Input: part model. Units: mm. Frame: model coordinates. Face numbers are marked on the shaded views. A direction names the side the tool comes from. Coordinates: 2 decimals unless noted, no trailing zeros. Loops run counter-clockwise (first coordinate to the right, second up) from the corner with the lowest first, then second, coordinate; pieces in that order, holes last. Notation, with made-up numbers: (29, 13.25) - (62, 13.25) arc R22 ccw to (62, 35.25) - close; hole circle Ø11 at (0.5, 8). An arc over 180 degrees is marked (long way). Use one line per item in the form item = value.
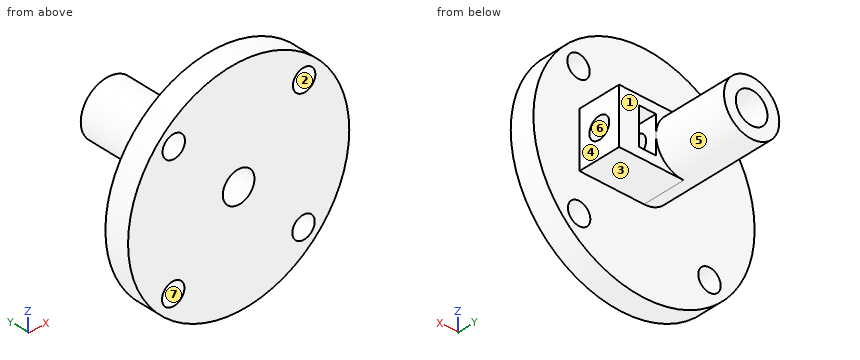
from build123d import *

# Parameters (mm, degrees)
SKETCH1_R           = 18
BOSS_EXTRUDE1_DEPTH = 4
SKETCH2_R           = 1.825
SKETCH2_R_2         = 2.575
CUT_EXTRUDE1_DEPTH  = 26.768197453
BOSS_EXTRUDE2_START = 19
SKETCH3_R           = 4.5
SKETCH3_R_2         = 2.575
BOSS_EXTRUDE2_DEPTH = 19
BOSS_EXTRUDE4_START = 7
BOSS_EXTRUDE4_DEPTH = 7
BOSS_EXTRUDE5_DEPTH = 7
SKETCH6_R           = 1.75
CUT_EXTRUDE2_DEPTH  = 10


with BuildPart() as part:
    # Sketch1 → Boss-Extrude1 (new body)
    with BuildSketch(Plane(origin=(0, 0, 0), x_dir=(1, 0, 0), z_dir=(0, 1, 0))):
        with Locations(Location((0, 0, 0), (0, 0, 270))):
            Circle(SKETCH1_R)
    extrude(amount=BOSS_EXTRUDE1_DEPTH)

    # Sketch2 → Cut-Extrude1 (cut, through all)
    with BuildSketch(Plane(origin=(0, 4, 0), x_dir=(1, 0, 0), z_dir=(0, 1, 0))):
        with Locations(Location((-10.654011001, 10.558979572, 0), (0, 0, 270))):
            Circle(SKETCH2_R)
        with Locations(Location((10.558979572, 10.654011001, 0), (0, 0, 270))):
            Circle(SKETCH2_R)
        with Locations(Location((10.654011001, -10.558979572, 0), (0, 0, 270))):
            Circle(SKETCH2_R)
        with Locations(Location((0, 0, 0), (0, 0, 270))):
            Circle(SKETCH2_R_2)
        with Locations(Location((-10.558979572, -10.654011001, 0), (0, 0, 270))):
            Circle(SKETCH2_R)
    extrude(amount=-CUT_EXTRUDE1_DEPTH, mode=Mode.SUBTRACT)

    # Sketch3 → Boss-Extrude2 (add)
    with BuildSketch(Plane(origin=(0, 4, 0), x_dir=(1, 0, 0), z_dir=(0, 1, 0)).offset(BOSS_EXTRUDE2_START)):
        with Locations(Location((0, 0, 0), (0, 0, 270))):
            Circle(SKETCH3_R)
        with Locations(Location((0, 0, 0), (0, 0, 270))):
            Circle(SKETCH3_R_2, mode=Mode.SUBTRACT)
    extrude(amount=-BOSS_EXTRUDE2_DEPTH)

    # Sketch3_4 → Boss-Extrude4 (add)
    with BuildSketch(Plane(origin=(0, 4, 0), x_dir=(1, 0, 0), z_dir=(0, 1, 0)).offset(BOSS_EXTRUDE4_START)):
        with BuildLine():
            ThreePointArc((0, 4.5), (3.181980515, 3.181980515), (4.5, 0))
            Line((4.5, 0), (4.5, 3))
            Line((4.5, 3), (4.5, 4.5))
            Line((4.5, 4.5), (0, 4.5))
        make_face()
        with BuildLine():
            Line((4.5, -3), (4.5, 0))
            ThreePointArc((4.5, 0), (3.181980515, -3.181980515), (0, -4.5))
            Line((0, -4.5), (4.5, -4.5))
            Line((4.5, -4.5), (4.5, -3))
        make_face()
    extrude(amount=-BOSS_EXTRUDE4_DEPTH)

    # Sketch3_5 → Boss-Extrude5 (add)
    with BuildSketch(Plane(origin=(0, 4, 0), x_dir=(1, 0, 0), z_dir=(0, 1, 0))):
        Polygon((4.5, 4.5), (4.5, 3), (7.26, 3), (7.26, -3), (4.5, -3), (4.5, -4.5), (10.5, -4.5), (10.5, 4.5), align=None)
    extrude(amount=BOSS_EXTRUDE5_DEPTH)

    # Sketch6 → Cut-Extrude2 (cut)
    with BuildSketch(Plane(origin=(10.5, 0, 0), x_dir=(0, 0, -1), z_dir=(1, 0, 0))):
        with Locations((0, 7.5)):
            Circle(SKETCH6_R)
    extrude(amount=-CUT_EXTRUDE2_DEPTH, mode=Mode.SUBTRACT)


solid = part.part
Q1. First-contact query: P1, Ø7.5, axis at y = 9, z = 0.5, coming from the +X side; P2, Ø1.4, axis at x = 5.5, y = 8, coming from the +Z side; P3, Ø6, axis at x = -10.65, z = -10.56, coming from the +Y side; P4, Ø3, axis at x = 0, z = 0, coming from the -Y side. Flat tips, straight axial feed; report the tip coordinate or a pass-through.
Check values:
P1 = 10.5
P2 = 4.5
P3 = 4
P4 = through
Q2. Cut plane A-A, the plane y = 7.5. Return loops of the section in (x, z) (3 decimals), then the cut area to 3 significant figures.
Check values:
outline = (0, -4.5) - (10.5, -4.5) - (10.5, -1.75) - (7.26, -1.75) - (7.26, -3) - (4.5, -3) - (4.5, -1.75) - (1.889, -1.75) arc R2.575 cw (long way) to (1.889, 1.75) - (4.5, 1.75) - (4.5, 3) - (7.26, 3) - (7.26, 1.75) - (10.5, 1.75) - (10.5, 4.5) - (0, 4.5) arc R4.5 ccw to start
area = 70.1 mm²
Q3. Cut plane C-C, the plane y = 17.5. Return loops of the section in (x, z) (3 decimals).
Check values:
outline = circle Ø9 at (0, 0); hole circle Ø5.15 at (0, 0)
Q4. Cut plane D-D, the plane z = 5.5. Return loops of the section in (x, y).
Check values:
outline = (-17.14, 0) - (17.14, 0) - (17.14, 4) - (-17.14, 4) - close
Q5. Set-up query: the marked faces 4, 5, 6 and 7. Return all of +Z, -Z, +X, -X, +Y, -Y with unobstructed straight access to the full face (end or side cutting, diameter ignored); none if empty.
Check values:
face_4 = +Z, -Z, +X, +Y
face_5 = +Y
face_6 = +X
face_7 = +Y, -Y
Q6. Ray query, line 1 along Z through (x, y) = (3.2, 7.5); line 2 along X through (y, z) = (9.25, 1); line 3 along Z through (x, y) = (3, 5.25). Return the intervals inside material, ascending. Write a range as [from, to].
Check values:
line_1 = [-4.5, -1.75], [1.75, 4.5]
line_2 = [-4.39, -2.37], [2.37, 4.5], [7.26, 10.5]
line_3 = [-4.5, 4.5]
Q7. Cut plane B-B, the plane x = -1. Return loops of the section in (y, z).
Check values:
outline = (0, -17.97) - (4, -17.97) - (4, -4.39) - (23, -4.39) - (23, -2.37) - (0, -2.37) - close; (0, 2.37) - (23, 2.37) - (23, 4.39) - (4, 4.39) - (4, 17.97) - (0, 17.97) - close
Q8. Pull-direction query (Z, two-part tool) for the marked faces 1, 2 and 3; classes: pulls with the +Z half, pulls with the -Z half, needs draft (parallel to the pull), parting line crosses it, or undercut.
Check values:
face_1 = needs draft
face_2 = undercut
face_3 = pulls with the -Z half
